```python
from build123d import *

# Parameters (mm, degrees)
F0_R     = 35
F1_DEPTH = 15
F2_W     = 35
F2_H     = 35
F3_DEPTH = 20
F4_W     = 20
F4_H     = 20
F5_DEPTH = 30


with BuildPart() as f1:
    # F0 (on Top) → F1 (new body)
    with BuildSketch(Plane.XY):
        Circle(F0_R)
    extrude(amount=F1_DEPTH)

    # F2 (on face) → F3 (join)
    with BuildSketch(Plane.XY.offset(15)):
        Rectangle(F2_W, F2_H)
    extrude(amount=F3_DEPTH)

    # F4 (on face) → F5 (join)
    with BuildSketch(Plane.XY.offset(35)):
        Rectangle(F4_W, F4_H)
    extrude(amount=F5_DEPTH)


solid = f1.part
```
Part model, mm, in its own coordinate system. A direction names the side the tool comes from. Round coordinates to 2 decimals unless told otherwise and drop trailing zeros. Write each loop counter-clockwise with the first axis right and the second up, starting at its lowest first coordinate (ties: lowest second). Pieces come first, ordered by that corner, then holes. Notation, with made-up numbers: (-13.75, 61.25) -> (20.25, 61.25) arc R21 ccw to (20.25, 95.25) -> close; hole circle Ø6 at (12, 87). An arc over 180 degrees is marked (long way). Return JSON: item names as keys, results as strings. Group by question number.
Q1. Saw through at C-C on z = 6. Write the cut outline in (x, y), plus the area to 3 significant figures.
Q2. Which spindle directions (+Z, -Z, +X, -X, +Y, -Y) get a long thin tool onto all of the face, cutting with end or side? Do faces 1 (the flat face through (-10, 0, 50)), 2 (the flat face through (0, -10, 50)), 3 (the flat face through (10, 0, 50)), 4 (the cylindrical face through (-28, -21, 7)), 5 (the flat face through (0, 17.5, 25)). Say none if no direction does.
Q3. Saw through at D-D on x = -12. Write the cut outline in (y, z), plus the area to 3 significant figures.
Q4. Pin check, flat tips, straight feed: pin 1 (10 mm diameter, centred on y = 2.5, z = 50, fed in from -X); pin 2 (10 mm diameter, centred on y = 5, z = 45, fed in from +X); pin 3 (22 mm diameter, centred on x = 2, z = 29.5, fed in from +Y); pin 4 (12 mm diameter, centred on x = -0.5, y = 0.5, fed in from -Z). Stop position of each tip, or through.
Q5. Probe L1, parallel to Z at x = -22.5, y = -5.5; L2, parallel to Y at x = -4, z = 43.5; L3, parallel to Z at x = 12.5, y = -4.5. List the from-to ranges inside material, lowest first. Write a range as [from, to].
Q6. Saw through at A-A on x = 0. Write the cut outline in (y, z), plus the area to 3 significant figures.
Answer:
{
 "1": {"outline": "circle Ø70 at (0, 0)", "area": "3,850 mm2"},
 "2": {"face 1": "+Z, -X, +Y, -Y", "face 2": "+Z, +X, -X, -Y", "face 3": "+Z, +X, +Y, -Y", "face 4": "+Z, -Z", "face 5": "+Z, +X, -X, +Y"},
 "3": {"outline": "(-32.88, 0) -> (32.88, 0) -> (32.88, 15) -> (17.5, 15) -> (17.5, 35) -> (-17.5, 35) -> (-17.5, 15) -> (-32.88, 15) -> close", "area": "1,690 mm2"},
 "4": {"pin 1": "x = -10", "pin 2": "x = 10", "pin 3": "y = 17.5", "pin 4": "z = 0"},
 "5": {"L1": "[0, 15]", "L2": "[-10, 10]", "L3": "[0, 35]"},
 "6": {"outline": "(-35, 0) -> (35, 0) -> (35, 15) -> (17.5, 15) -> (17.5, 35) -> (10, 35) -> (10, 65) -> (-10, 65) -> (-10, 35) -> (-17.5, 35) -> (-17.5, 15) -> (-35, 15) -> close", "area": "2,350 mm2"}
}
